Source: CAD feature listing. Evaluate the final solid. Frame: model axes, mm. Face numbers are marked on the shaded views. A direction names the side the tool comes from. Round coordinates to 2 decimals unless told otherwise and drop trailing zeros. Order: outer loops, then holes, each group sorted by start corner. A loop starts at its lowest first (then second) coordinate and runs counter-clockwise, first axis right, second up. Notation, with made-up numbers: (50, 14.5) - (102, 14.5) arc R12 cw to (102, 20.5) - close; hole circle Ø10 at (78, 57). An arc over 180 degrees is marked (long way). Use one line per item in the form item = value. Start each with the question number.
Q1. Ray query, line 1 (X direction, y = 6.5, z = 0) (3 decimals); line 2 (X direction, y = 4, z = 0.75); line 3 (Z direction, x = 0.15, y = 2.75). Return the intervals inside material, ascending. Write a range as [from, to].
Q2. Cut plane C-C, the plane y = 3.5. Return the cut outline in (x, z) (3 decimals), and give its area (3 significant figures).
Q3. Cut plane B-B, the plane z = 0. Return the cut outline in (x, y) (3 decimals).
Q4. Set-up query: the marked faces 1 and 2. Return all of +Z, -Z, +X, -X, +Y, -Y with unobstructed straight access to the full face (end or side cutting, diameter ignored); none if empty.
Q5. Cut plane A-A, the plane x = 0. Return the cut outline in (y, z) (3 decimals), and give its area (3 significant figures).
Q6. Cut plane D-D, the plane y = 1. Return the cut outline in (x, z).
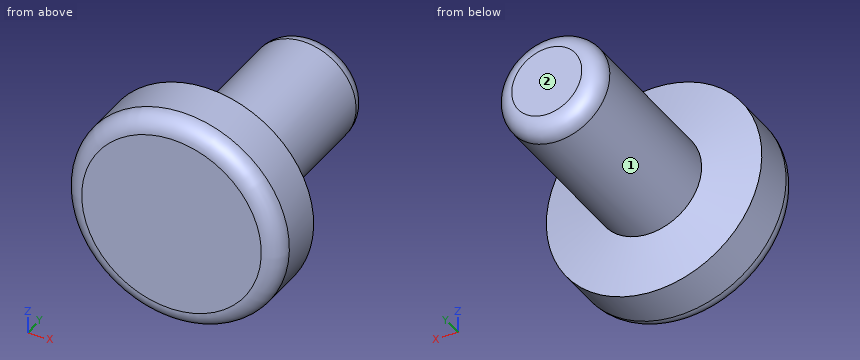
from build123d import *

# Parameters (mm, degrees)
CROQUIS1_R              = 3
SALIENTE_EXTRUIR1_DEPTH = 2
CROQUIS2_R              = 1.475
SALIENTE_EXTRUIR2_DEPTH = 5
CHAFL_N1_SIZE           = 0.3
CHAFL_N1_SIZE_2         = 1.701384546
REDONDEO1_R             = 0.5
REDONDEO2_R             = 0.5


with BuildPart() as part:
    # Croquis1 → Saliente-Extruir1 (new body)
    with BuildSketch(Plane(origin=(0, 0, 0), x_dir=(1, 0, 0), z_dir=(0, 1, 0))):
        with Locations(Location((0, 0, 0), (0, 0, 270))):
            Circle(CROQUIS1_R)
    extrude(amount=SALIENTE_EXTRUIR1_DEPTH)

    # Croquis2 → Saliente-Extruir2 (add)
    with BuildSketch(Plane(origin=(0, 2, 0), x_dir=(1, 0, 0), z_dir=(0, 1, 0))):
        with Locations(Location((0, 0, 0), (0, 0, 270))):
            Circle(CROQUIS2_R)
    extrude(amount=SALIENTE_EXTRUIR2_DEPTH)

    # Chaflán1
    # the kernel refuses this chamfer: 1.701384546, 0.3 mm, written as the material it takes off along each edge
    with BuildSketch(Plane(origin=(0, 2, 0), x_dir=(0, 0, 1), z_dir=(-1, 0, 0))) as chafl_n1_piece_1_section:
        Polygon((3, -CHAFL_N1_SIZE), (3 - CHAFL_N1_SIZE_2, 0), (3, 0), align=None)
    chafl_n1_piece_1 = revolve(axis=Axis((0, 2, 0), (0, 1, 0)), mode=Mode.PRIVATE)
    chafl_n1_piece_1 = chafl_n1_piece_1 - Plane(origin=(0, 1.84524898, 0), x_dir=(0, 0, 1), z_dir=(0, -1, 0)) * Cylinder(1.475, 12, mode=Mode.PRIVATE)
    add(chafl_n1_piece_1, mode=Mode.SUBTRACT)

    # Redondeo1
    redondeo1_edges = [part.edges().sort_by_distance(p)[0] for p in [
        (0, 7, -1.475),
    ]]
    fillet(redondeo1_edges, radius=REDONDEO1_R)

    # Redondeo2
    redondeo2_edges = [part.edges().sort_by_distance(p)[0] for p in [
        (0, 0, -3),
    ]]
    fillet(redondeo2_edges, radius=REDONDEO2_R)


solid = part.part
Completed:
q1.line_1 = [-1.475, 1.475]
q1.line_2 = [-1.27, 1.27]
q1.line_3 = [-1.47, 1.47]
q2.outline = circle Ø2.95 at (0, 0)
q2.area = 6.83 mm2
q3.outline = (-3, 0.5) arc R0.5 ccw to (-2.5, 0) - (2.5, 0) arc R0.5 ccw to (3, 0.5) - (3, 1.7) - (1.475, 1.969) - (1.475, 6.5) arc R0.5 ccw to (0.975, 7) - (-0.975, 7) arc R0.5 ccw to (-1.475, 6.5) - (-1.475, 1.969) - (-3, 1.7) - close
q4.face_1 = +Y
q4.face_2 = +Z, -Z, +X, -X, +Y
q5.outline = (0, -2.5) arc R0.5 ccw to (0.5, -3) - (1.7, -3) - (1.969, -1.475) - (6.5, -1.475) arc R0.5 ccw to (7, -0.975) - (7, 0.975) arc R0.5 ccw to (6.5, 1.475) - (1.969, 1.475) - (1.7, 3) - (0.5, 3) arc R0.5 ccw to (0, 2.5) - close
q5.area = 26.0 mm2
q6.outline = circle Ø6 at (0, 0)
